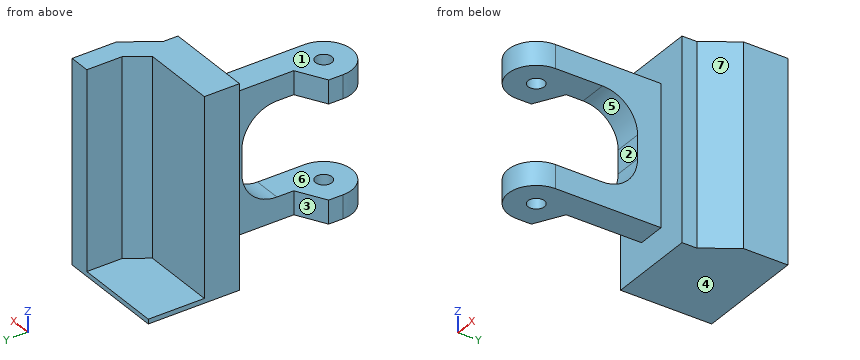
```python
from build123d import *

# Parameters (mm, degrees)
ESQUISSE1_R        = 3.5
BOSS_EXTRU_1_DEPTH = 10
BOSS_EXTRU_2_DEPTH = 5
ESQUISSE3_W        = 12
ESQUISSE3_H        = 40
BOSS_EXTRU_3_DEPTH = 5
CONG_1_R           = 15
ESQUISSE4_W        = 38
ESQUISSE4_H        = 86
BOSS_EXTRU_4_DEPTH = 15
BOSS_EXTRU_5_DEPTH = 85
BOSS_EXTRU_6_DEPTH = 2


with BuildPart() as part:
    # Esquisse1 → Boss.-Extru.1 (new body)
    with BuildSketch(Plane.XY):
        with BuildLine():
            Line((-12, 0), (-12, 6.188999999))
            Line((-12, 6.188999999), (0, 12.795952069))
            Line((0, 12.795952069), (0, 40))
            Line((0, 40), (12, 40))
            Line((12, 40), (12, 0))
            ThreePointArc((12, 0), (0, -12), (-12, 0))
        make_face()
        Circle(ESQUISSE1_R, mode=Mode.SUBTRACT)
    extrude(amount=BOSS_EXTRU_1_DEPTH)


with BuildPart() as body_2:
    # Esquisse2 → Boss.-Extru.2 (new body)
    with BuildSketch(Plane(origin=(0, 40, 0), x_dir=(1, 0, 0), z_dir=(0, 1, 0))):
        Polygon((0, -10), (0, -60), (12, -60), (12, -10), (12, 0), (0, 0), align=None)
    extrude(amount=BOSS_EXTRU_2_DEPTH)


with BuildPart() as body_3:
    # Symétrie2: mirrored copy
    add(part.part.mirror(Plane.XY.offset(30)))

    # Combiner1: union body 2, part
    add(body_2.part)
    add(part.part)

    # Esquisse3 → Boss.-Extru.3 (add)
    with BuildSketch(Plane.XZ.offset(-40)):
        with Locations((6, 30)):
            Rectangle(ESQUISSE3_W, ESQUISSE3_H)
    extrude(amount=BOSS_EXTRU_3_DEPTH)

    # Congé1
    cong_1_edges = [body_3.edges().sort_by_distance(p)[0] for p in [
        (6, 35, 10),
        (6, 35, 50),
    ]]
    fillet(cong_1_edges, radius=CONG_1_R)

    # Esquisse4 → Boss.-Extru.4 (add)
    with BuildSketch(Plane(origin=(0, 45, 0), x_dir=(1, 0, 0), z_dir=(0, 1, 0))):
        with Locations((6, -30)):
            Rectangle(ESQUISSE4_W, ESQUISSE4_H)
    extrude(amount=BOSS_EXTRU_4_DEPTH)

    # Esquisse5 → Boss.-Extru.5 (add)
    with BuildSketch(Plane.XY.offset(73)):
        Polygon((25, 51.312184347), (34.08898267, 64.966903238), (34.08898267, 83.946962496), (25, 83.946962496), (25, 68.926771716), (19.136954754, 60), align=None)
    extrude(amount=-BOSS_EXTRU_5_DEPTH)

    # Esquisse6 → Boss.-Extru.6 (add)
    with BuildSketch(Plane(origin=(0, 0, -13), x_dir=(-1, 0, 0), z_dir=(0, 0, -1))):
        Polygon((-34.08898267, 64.966903238), (-25, 51.312184347), (-25, 45), (13, 45), (13, 60), (13, 83.946962496), (-25, 83.946962496), (-34.08898267, 83.946962496), align=None)
    extrude(amount=-BOSS_EXTRU_6_DEPTH)


solid = body_3.part
```
Input: part model. Units: mm. Frame: model coordinates. Face numbers are marked on the shaded views. A direction names the side the tool comes from. Give positions to 0.01 mm unless a question says otherwise; leave off trailing zeros. Loops run counter-clockwise (first coordinate to the right, second up) from the corner with the lowest first, then second, coordinate; pieces in that order, holes last.
1) Contact query for flat-ended pins moving along their axis: pin 1 (5.5 mm diameter, centred on x = 0, y = 0, fed in from -Z); pin 2 (7 mm diameter, centred on y = 3.5, z = 3, fed in from -X); pin 3 (1.5 mm diameter, centred on x = 3, z = 32, fed in from -Y); pin 4 (7 mm diameter, centred on x = -0.5, y = 8, fed in from +Z). Output: stop coordinate, or through.
A:
pin 1: passes through
pin 2: stops at x = -12
pin 3: stops at y = 35
pin 4: stops at z = 60
2) Line query: L1, parallel to Z at x = 5, y = 0; L2, parallel to X at y = 47, z = -3; L3, parallel to X at y = 35.5, z = 40. Output: solid intervals per line, ascending.
A:
L1: z = 0 to 10, 50 to 60
L2: x = -13 to 25
L3: x = 0 to 12
3) Section query A-A on x = 14.5. Return the cut outline in (y, z).
A:
outline: (45, -13) - (83.95, -13) - (83.95, -11) - (60, -11) - (60, 73) - (45, 73) - close
4) Section query C-C on x = -6.5. Return the cut outline in (y, z).
A:
outline: (-10.09, 0) - (9.22, 0) - (9.22, 10) - (-10.09, 10) - close; (-10.09, 50) - (9.22, 50) - (9.22, 60) - (-10.09, 60) - close; (45, -13) - (83.95, -13) - (83.95, -11) - (60, -11) - (60, 73) - (45, 73) - close
5) Mould query, pull axis Z, two halves, no side actions, for the marked faces 4, 5, 6 and 7. Classes: released by +Z, released by -Z, zero draft, split by the parting line, or undercut.
A:
face 4: released by -Z
face 5: undercut
face 6: undercut
face 7: zero draft
6) Section query B-B on z = 47. Return the cut outline in (x, y), and give its area (3 significant figures).
A:
outline: (-13, 45) - (0, 45) - (0, 29) - (12, 29) - (12, 45) - (25, 45) - (25, 51.31) - (34.09, 64.97) - (34.09, 83.95) - (25, 83.95) - (25, 68.93) - (19.14, 60) - (-13, 60) - close
area: 1,020 mm2
7) Reachability of the marked faces 1, 2 and 3 from +Z, -Z, +X, -X, +Y, -Y: full face, straight path, thin tool, end or side. Return the list, or none.
A:
face 1: +Z, +X, -X, -Y
face 2: +X, -X, -Y
face 3: +Z, -Z, -X
8) Section query D-D on y = 77. Return the cut outline in (x, z), and give its area (3 significant figures).
A:
outline: (-13, -13) - (34.09, -13) - (34.09, 73) - (25, 73) - (25, -11) - (-13, -11) - close
area: 858 mm2
